Autodesk Inventor part; units mm, degrees
ref_plane "YZ Plane" through (0, 0, 0) normal (1, 0, 0) x (0, 1, 0)
ref_plane "XZ Plane" through (0, 0, 0) normal (0, 1, 0) x (-1, 0, 0)
ref_plane "XY Plane" through (0, 0, 0) normal (0, 0, 1) x (1, 0, 0)
sketch "Sketch1" plane through (0, 0, 0) normal (0, 0, 1) x (1, 0, 0)
  arc A0 (-13.4919, 42.7251) -> (-13.4919, -20.7749) centre (-13.4919, 10.9751) ccw
  arc A1 (94.4581, -20.7749) -> (94.4581, 42.7251) centre (94.4581, 10.9751) ccw
  line L0 (-13.4919, 42.7251) -> (94.4581, 42.7251)
  line L1 (94.4581, -20.7749) -> (-13.4919, -20.7749)
  line L2 (94.4581, 44.3126) -> (-13.4919, 44.3126)
  arc A2 (-13.4919, 44.3126) -> (-13.4919, -22.3624) centre (-13.4919, 10.9751) ccw
  line L3 (-13.4919, -22.3624) -> (94.4581, -22.3624)
  arc A3 (94.4581, -22.3624) -> (94.4581, 44.3126) centre (94.4581, 10.9751) ccw
  point P0 (0, 0)
  dimension "d2" = 31.75
  dimension "d3" = 107.95
  dimension "d4" = 1.5875
extrude "Extrusion1" add sketch "Sketch1" along normal blind 50.8
equation "\"d2\" = d1"
equation "\"d3\" = d0"
equation "\"d0\" = 107.95"
equation "\"d1\" = 31.75"
properties part number "Polyurethane Belt STOCK" material "Rubber"
Input: part model. Units: mm. Frame: model coordinates. A direction names the side the tool comes from. Coordinates: 2 decimals unless noted, no trailing zeros. Loops run counter-clockwise (first coordinate to the right, second up) from the corner with the lowest first, then second, coordinate; pieces in that order, holes last.
Q1. Material intervals for line 1 (Y direction, x = 57.5, z = 39); line 2 (X direction, y = 22, z = 15); line 3 (Y direction, x = -33.5, z = 29), sorted ascending.
Q2. Cut plane C-C (y = 31.5). Output: boundary loops of the cut face in (x, z).
Q3. Draft query along Y for faces 3 (the face through (40, 42.725, 25)), 4 (the face through (41, 44.313, 25)), 5 (the face through (40, 43, 50.8)), 6 (the face through (-45.234, 10.277, 25.044)). Return one class per face: +Y half, -Y half, draft (parallel to the pull), parting line (faces both ways), or undercut.
Q4. Contact query for flat-ended pins moving along their axis: pin 1 (4 mm diameter, centred on y = 11, z = 7.5, fed in from -X); pin 2 (5 mm diameter, centred on y = 26, z = 25, fed in from -X); pin 3 (1 mm diameter, centred on y = 34.5, z = 27, fed in from +X). Output: stop coordinate, or through.
Q5. Set-up query: faces 1 (the face through (40, 43, 0)), 2 (the face through (126.2, 11.7, 25)). Return all of +Z, -Z, +X, -X, +Y, -Y with unobstructed straight access to the full face (end or side cutting, diameter ignored); none if empty.
Q6. Cut plane A-A (x = 52). Output: boundary loops of the cut face in (y, z).
Working result:
1. line 1: y = -22.36 to -20.77, 42.73 to 44.31
1. line 2: x = -44.95 to -43.27, 124.23 to 125.92
1. line 3: y = -15.69 to -13.68, 35.63 to 37.64
2. outline: (-39.76, 0) - (-37.72, 0) - (-37.72, 50.8) - (-39.76, 50.8) - close; (118.68, 0) - (120.73, 0) - (120.73, 50.8) - (118.68, 50.8) - close
3. face 3: undercut
3. face 4: +Y half
3. face 5: draft
3. face 6: undercut
4. pin 1: stops at x = -46.83
4. pin 2: stops at x = -44.39
4. pin 3: stops at x = 118.57
5. face 1: -Z, +X, -X, +Y, -Y
5. face 2: +Z, -Z
6. outline: (-22.36, 0) - (-20.77, 0) - (-20.77, 50.8) - (-22.36, 50.8) - close; (42.73, 0) - (44.31, 0) - (44.31, 50.8) - (42.73, 50.8) - close
